```python
from build123d import *

# Parameters (mm, degrees)
BOSS_EXTRUDE1_DEPTH = 5
SKETCH4_R           = 3
CUT_EXTRUDE1_DEPTH  = 5
SKETCH6_R           = 0.17
CUT_EXTRUDE2_DEPTH  = 10.128709292
CHAMFER2_SIZE       = 0.875
CHAMFER2_SIZE2      = 2


with BuildPart() as part:
    # Sketch1 → Boss-Extrude1 (new body)
    with BuildSketch(Plane(origin=(0, 0, 0), x_dir=(1, 0, 0), z_dir=(0, 1, 0))):
        Polygon((5.773502692, 0), (2.886751346, 5), (-2.886751346, 5), (-5.773502692, 0), (-2.886751346, -5), (2.886751346, -5), align=None)
    extrude(amount=BOSS_EXTRUDE1_DEPTH)

    # Sketch3 → Revolve1 (revolve)
    with BuildSketch(Plane.XY):
        with BuildLine():
            Line((0, 5), (-4.5, 5))
            ThreePointArc((-4.5, 5), (-3.181980515, 8.181980515), (0, 9.5))
            Line((0, 9.5), (0, 5))
        make_face()
    revolve(axis=Axis((0, 0, 0), (0, 1, 0)))

    # Sketch4 → Cut-Extrude1 (cut)
    with BuildSketch(Plane.XZ):
        with Locations(Location((0, 0, 0), (0, 0, 270))):
            Circle(SKETCH4_R)
    extrude(amount=-CUT_EXTRUDE1_DEPTH, mode=Mode.SUBTRACT)

    # Sketch6 → Cut-Extrude2 (cut, through all)
    with BuildSketch(Plane.XZ.offset(-5)):
        with Locations(Location((0, 0, 0), (0, 0, 270))):
            Circle(SKETCH6_R)
    extrude(amount=-CUT_EXTRUDE2_DEPTH, mode=Mode.SUBTRACT)

    # Chamfer2
    chamfer2_edges = [part.edges().sort_by_distance(p)[0] for p in [
        (0, 5, 0.17),
    ]]
    chamfer2_side = [part.faces().sort_by_distance(p)[0] for p in [
        (0, 5, 2.915147186),
    ]]
    chamfer(chamfer2_edges, length=CHAMFER2_SIZE, length2=CHAMFER2_SIZE2, reference=chamfer2_side[0])


solid = part.part
```
Check sheet for the modelled part. Datum: model origin and axes. Units: mm. A direction names the side the tool comes from. Give positions to 0.01 mm unless a question says otherwise; leave off trailing zeros. Order: outer loops, then holes, each group sorted by start corner. A loop starts at its lowest first (then second) coordinate and runs counter-clockwise, first axis right, second up. Notation, with made-up numbers: M 81,62 L 113,62 A23 cw 113,72 Z; hole C 83.5,-0.75 d10. An arc over 180 degrees is marked long. Answer in a Markdown table with one row per item. Add a question column.
Q1. Sectioned sample at A-A, the plane x = 0. Record the boundary of the cut face in (y, z) (3 decimals).
Q2. Gauge pin test, flat ends, axial feed: pin 1 Ø2 at (x, z) = (-0.5, -0.5) entering from -Y; pin 2 Ø1.5 at (x, z) = (4.5, -1.5) entering from +Y; pin 3 Ø2 at (y, z) = (5.5, -4) entering from +X. Record the tip position at first contact, or that the pin passes through.
Q3. Access from +Z, -Z, +X, -X, +Y, -Y to the whole of each face (thin tool, end or side, straight path). Record for faces 1 (the flat face through (4.31, 2.465, 2.535)), 2 (the cylindrical face through (0.9, 2.46, -2.86)), 3 (the flat face through (3, 5, -4)).
Q4. Sectioned sample at C-C, the plane z = 3.25. Record the boundary of the cut face in (x, y), and give its area (3 significant figures).
Q5. Sectioned sample at D-D, the plane x = -4. Record the boundary of the cut face in (y, z).
Q6. Sectioned sample at B-B, the plane y = 2. Record the boundary of the cut face in (x, z), and give its area (3 significant figures).
Q7. Release check for a two-part mould opening along X. For faces 4 (the flat face through (-4.31, 2.465, -2.535)), 5 (the flat face through (0, 5, -1.3)), 6 (the flat face through (4.35, 2.465, -2.465)), 7 (the flat face through (0, 2, -5)) record: released by +X, released by -X, zero draft, split by the parting line, or undercut.
Q8. Thickness scan on L1, parallel to Y at x = -3, z = 4.75; L2, parallel to Z at x = 0, y = 8.2; L3, parallel to Z at x = 0, y = 8.55. Record the ranges inside material, lowest first.
Verdict:
| question | item | result |
|---|---|---|
| 1 | outline | M 0,-5 L 5,-5 L 5,-4.5 A4.5 ccw 9.497,-0.17 L 7,-0.17 L 5,-1.045 L 5,-3 L 0,-3 Z; M 0,3 L 5,3 L 5,1.045 L 7,0.17 L 9.497,0.17 A4.5 ccw 5,4.5 L 5,5 L 0,5 Z |
| 2 | pin 1 | y = 5 |
| 2 | pin 2 | y = 7.07 |
| 2 | pin 3 | x = 3.96 |
| 3 | face 1 | +Z, +X, +Y, -Y |
| 3 | face 2 | -Y |
| 3 | face 3 | +Y |
| 4 | outline | M -3.9,0 L 3.9,0 L 3.9,5 L 3.11,5 A3.11 ccw -3.11,5 L -3.9,5 Z |
| 4 | area | 54.2 mm² |
| 5 | outline | M 0,-3.07 L 5,-3.07 L 5,-2.06 A2.06 ccw 5,2.06 L 5,3.07 L 0,3.07 Z |
| 6 | outline | M -5.77,0 L -2.89,-5 L 2.89,-5 L 5.77,0 L 2.89,5 L -2.89,5 Z; hole C 0,0 d6 |
| 6 | area | 58.3 mm² |
| 7 | face 4 | released by -X |
| 7 | face 5 | undercut |
| 7 | face 6 | released by +X |
| 7 | face 7 | zero draft |
| 8 | L1 | 0 to 5 |
| 8 | L2 | -3.16 to -0.17, 0.17 to 3.16 |
| 8 | L3 | -2.77 to -0.17, 0.17 to 2.77 |
